from build123d import *

# Parameters (mm, degrees)
M4_START                = 35.5
SKETCH1_R               = 2
M4_SHANK_AND_GRIP_DEPTH = 29.5
HEAD_START              = 61.6
SKETCH2_R               = 3.4
HEAD_DEPTH              = 3.4
LOCKNUT_START           = 35.5
SKETCH3_R               = 3.4
LOCKNUT_DEPTH           = 2.9


with BuildPart() as part:
    # Sketch1 → M4 shank and grip (new body)
    with BuildSketch(Plane.XY.offset(M4_START)):
        Circle(SKETCH1_R)
    extrude(amount=M4_SHANK_AND_GRIP_DEPTH)

    # Sketch2 → Head (add)
    with BuildSketch(Plane.XY.offset(HEAD_START)):
        Circle(SKETCH2_R)
    extrude(amount=HEAD_DEPTH)

    # Sketch3 → Locknut (add)
    with BuildSketch(Plane.XY.offset(LOCKNUT_START)):
        Circle(SKETCH3_R)
    extrude(amount=LOCKNUT_DEPTH)


solid = part.part
The model under review builds one solid part; all positions refer to its coordinate system, in mm. A direction names the side the tool comes from. Coordinates: 2 decimals unless noted, no trailing zeros. Loops run counter-clockwise (first coordinate to the right, second up) from the corner with the lowest first, then second, coordinate; pieces in that order, holes last. Notation, with made-up numbers: (82.5, 54.5) -> (137.5, 54.5) arc R24 cw to (137.5, 84.5) -> close; hole circle Ø7 at (14.25, 49). An arc over 180 degrees is marked (long way). Use a Markdown table: item, result. Add a question column.
1. Add section C-C on y = 2.75. Write out the cut boundary in (x, z), plus the area to 3 significant figures.
2. Machinability: for faces 4 (the face through (-0.74, -3.32, 63.28)), 5 (the face through (0, -2, 50)), which of the approach directions +Z, -Z, +X, -X, +Y, -Y give a long, thin tool a straight path to every point of the face, cutting with its end or side? Answer none if there is none.
3. Add section D-D on z = 54.5. Write out the cut boundary in (x, y).
4. Draft analysis for pull direction Z (two halves, no side actions). For faces 1 (the face through (-0.74, -3.32, 36.93)), 2 (the face through (0, -2.2, 38.4)), 3 (the face through (0, 0, 65)), state which applies: pulls with the +Z half, pulls with the -Z half, needs draft (parallel to the pull), parting line crosses it, or undercut.
5. Clearance check with a flat-ended pin moving along its axis: pin 1 Ø1 at (y, z) = (1, 50.5) entering from +X. State where the tip first meets the part, or that it passes through.
6. To check wall thickness, follow line 1 (Z direction, x = 2.25, y = 2); line 2 (X direction, y = 0, z = 40.5); line 3 (X direction, y = 1.75, z = 59.5). State the ranges of each line that lie inside material, in increasing order.
7. Add section A-A on x = 0. Write out the cut boundary in (y, z).
Returned:
| question | item | result |
|---|---|---|
| 1 | outline | (-2, 35.5) -> (2, 35.5) -> (2, 38.4) -> (-2, 38.4) -> close; (-2, 61.6) -> (2, 61.6) -> (2, 65) -> (-2, 65) -> close |
| 1 | area | 25.2 mm² |
| 2 | face 4 | +Z, -Z |
| 2 | face 5 | none |
| 3 | outline | circle Ø4 at (0, 0) |
| 4 | face 1 | needs draft |
| 4 | face 2 | undercut |
| 4 | face 3 | pulls with the +Z half |
| 5 | pin 1 | stops at x = 1.94 |
| 6 | line 1 | z = 35.5 to 38.4, 61.6 to 65 |
| 6 | line 2 | x = -2 to 2 |
| 6 | line 3 | x = -0.97 to 0.97 |
| 7 | outline | (-3.4, 35.5) -> (3.4, 35.5) -> (3.4, 38.4) -> (2, 38.4) -> (2, 61.6) -> (3.4, 61.6) -> (3.4, 65) -> (-3.4, 65) -> (-3.4, 61.6) -> (-2, 61.6) -> (-2, 38.4) -> (-3.4, 38.4) -> close |
